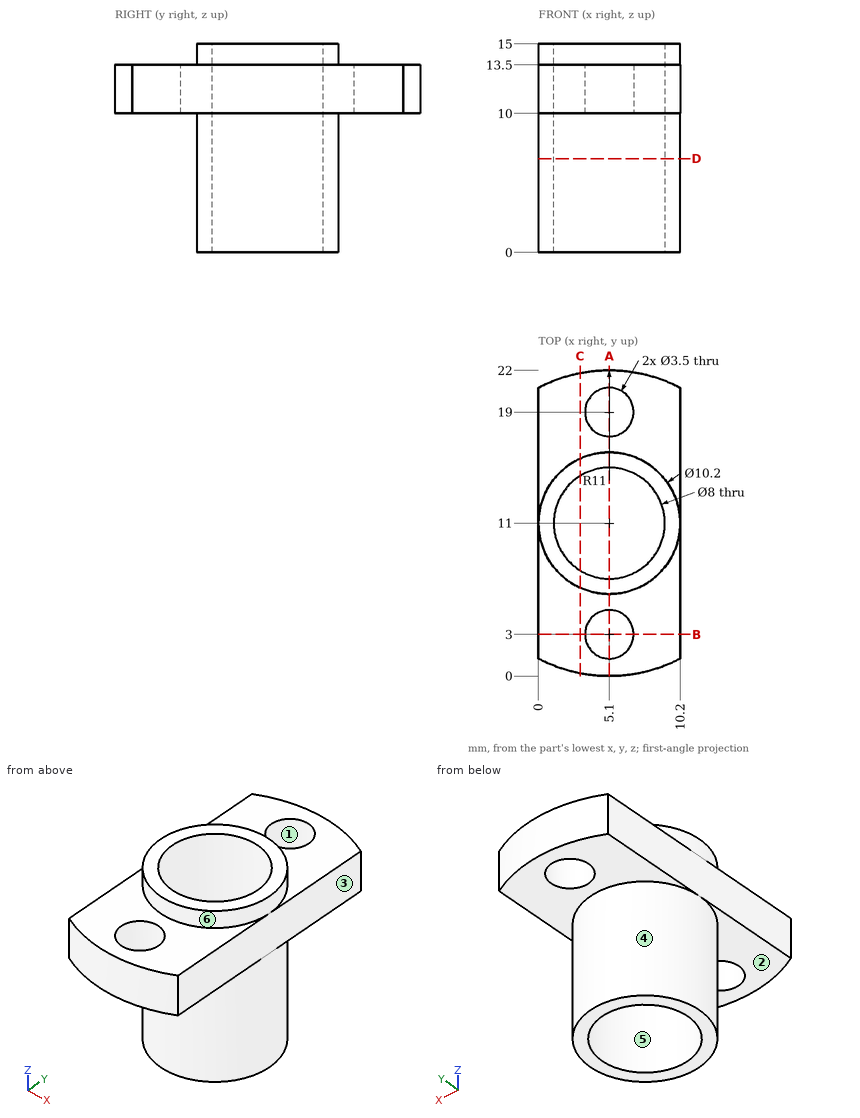
The drawing under review shows one solid part. Ordinate dimensions are in mm from its lowest x, y, z. A direction names the side the tool comes from. Coordinates: 2 decimals unless noted, no trailing zeros. Order: outer loops, then holes, each group sorted by start corner. A loop starts at its lowest first (then second) coordinate and runs counter-clockwise, first axis right, second up. Notation, with made-up numbers: (26, -3.5) -> (34, -3.5) arc R30 cw to (34, 29.5) -> close; hole circle Ø10 at (-36.5, 59). An arc over 180 degrees is marked (long way). Answer as CSV lines item,"result".
Q1. For the marked faces 5 and 6, list the 3-axis set-ups (+Z, -Z, +X, -X, +Y, -Y) from which the entire face can be reached by the end or side of a thin tool; tool diameter is ignored.
Model answer:
face 5,"+Z, -Z"
face 6,"+Z"
Q2. We need section D-D (z = 6.75). State the section outline as (x, y) points, plus the area to 3 significant figures.
Model answer:
outline,"circle Ø10.2 at (5.1, 11); hole circle Ø8 at (5.1, 11)"
area,"31.4 mm2"
Q3. Draft analysis for pull direction X (two halves, no side actions). For the marked faces 1, 2, 3 and 4, state which applies: released by +X, released by -X, zero draft, split by the parting line, or undercut.
Model answer:
face 1,"undercut"
face 2,"zero draft"
face 3,"released by +X"
face 4,"split by the parting line"
Q4. Clearance check with flat-ended pins moving along their axes: pin 1 Ø4 at (x, y) = (5.1, 19) entering from -Z; pin 2 Ø3 at (x, z) = (2.5, 5.5) entering from +Y; pin 3 Ø3 at (x, y) = (3.5, 4) entering from +Z. State where each tip first meets the part, or that it passes through.
Model answer:
pin 1,"stops at z = 10"
pin 2,"stops at y = 15.98"
pin 3,"stops at z = 13.5"
Q5. Wall thickness on line 1 along Y through (x, z) = (5.1, 10.8); line 2 along Z through (x, y) = (3.25, 4); line 3 along Y through (x, z) = (7.25, 7.75): over which ranges is each line inside the solid? List them lowest first. Write a range as [from, to].
Model answer:
line 1,"y = [0, 1.25], [4.75, 7], [15, 17.25], [20.75, 22]"
line 2,"z = [10, 13.5]"
line 3,"y = [6.38, 7.63], [14.37, 15.62]"
Q6. We need section A-A (x = 5.1). State the section outline as (y, z) points.
Model answer:
outline,"(0, 10) -> (1.25, 10) -> (1.25, 13.5) -> (0, 13.5) -> close; (4.75, 10) -> (5.9, 10) -> (5.9, 0) -> (7, 0) -> (7, 15) -> (5.9, 15) -> (5.9, 13.5) -> (4.75, 13.5) -> close; (15, 0) -> (16.1, 0) -> (16.1, 10) -> (17.25, 10) -> (17.25, 13.5) -> (16.1, 13.5) -> (16.1, 15) -> (15, 15) -> close; (20.75, 10) -> (22, 10) -> (22, 13.5) -> (20.75, 13.5) -> close"
Q7. We need section C-C (x = 3). State the section outline as (y, z) points, plus the area to 3 significant figures.
Model answer:
outline,"(0.2, 10) -> (6.35, 10) -> (6.35, 0) -> (7.6, 0) -> (7.6, 15) -> (6.35, 15) -> (6.35, 13.5) -> (0.2, 13.5) -> close; (14.4, 0) -> (15.65, 0) -> (15.65, 10) -> (21.8, 10) -> (21.8, 13.5) -> (15.65, 13.5) -> (15.65, 15) -> (14.4, 15) -> close"
area,"80.3 mm2"
Q8. We need section B-B (y = 3). State the section outline as (x, z) points.
Model answer:
outline,"(0, 10) -> (3.35, 10) -> (3.35, 13.5) -> (0, 13.5) -> close; (6.85, 10) -> (10.2, 10) -> (10.2, 13.5) -> (6.85, 13.5) -> close"
